```python
from build123d import *

# Parameters (mm, degrees)
SKETCH1_R           = 6.5
BOSS_EXTRUDE1_DEPTH = 8.000000002
SKETCH2_R           = 5
CUT_EXTRUDE1_DEPTH  = 5.999999938


with BuildPart() as part:
    # Sketch1 → Boss-Extrude1 (new body)
    with BuildSketch(Plane(origin=(0, 0, 0), x_dir=(1, 0, 0), z_dir=(0, 1, 0))):
        Circle(SKETCH1_R)
        with BuildLine():
            ThreePointArc((6.5, 0), (5.252972745, -3.828351779), (1.990376203, -6.187762323))
            Line((1.990376203, -6.187762323), (12.348635171, -2.855890303))
            ThreePointArc((12.348635171, -2.855890303), (14.43, 0), (12.348635171, 2.855890303))
            Line((12.348635171, 2.855890303), (1.990376203, 6.187762323))
            ThreePointArc((1.990376203, 6.187762323), (5.252972745, 3.828351779), (6.5, 0))
        make_face()
    extrude(amount=BOSS_EXTRUDE1_DEPTH)

    # Sketch2 → Cut-Extrude1 (cut)
    with BuildSketch(Plane(origin=(0, 8.000000002, 0), x_dir=(1, 0, 0), z_dir=(0, 1, 0))):
        with Locations(Location((0, 0, 0), (0, 0, 270))):
            Circle(SKETCH2_R)
    extrude(amount=-CUT_EXTRUDE1_DEPTH, mode=Mode.SUBTRACT)


solid = part.part
```
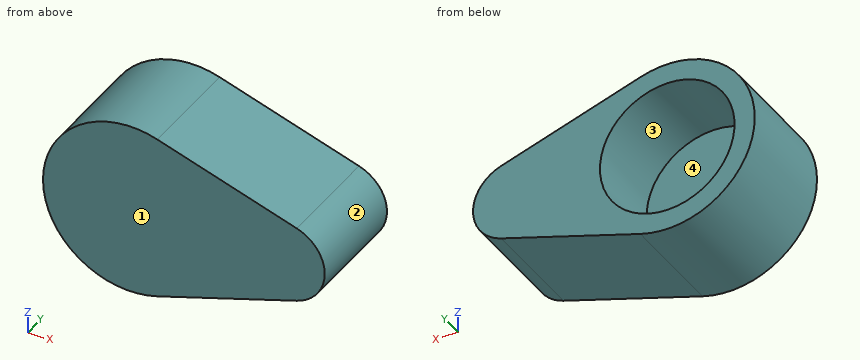
CAD build for the part. Positions are in the model's coordinates, mm. Face numbers are marked on the shaded views. Coordinates: 2 decimals unless noted, no trailing zeros. Write each loop counter-clockwise with the first axis right and the second up, starting at its lowest first coordinate (ties: lowest second). Pieces come first, ordered by that corner, then holes. Notation, with made-up numbers: (-36, 70) -> (-5, 70) arc R20 ccw to (-5, 95) -> close; hole circle Ø6 at (49.25, -26). An arc over 180 degrees is marked (long way). Return JSON: item names as keys, results as strings. Group by question number.
Q1. Flat gauge pins, fed straight in: pin 1 (1 mm diameter, centred on x = 6, z = 0.5, fed in from -Y); pin 2 (2 mm diameter, centred on x = -3, y = 4.5, fed in from +Z); pin 3 (1.5 mm diameter, centred on y = 6.5, z = -3.5, fed in from -X); pin 4 (1.5 mm diameter, centred on y = 3.5, z = 1.5, fed in from +X). Where does each tip first touch, or does it go through?
Q2. Cut at D-D, the plane z = 5.25. Give the cut face in (x, y), then the cut area to 3 significant figures.
Q3. Pull direction Z, two halves, no side cores. Call the marked faces 1, 2, 3 and 4: released by +Z, released by -Z, zero draft, split by the parting line, or undercut.
Q4. Drill centre lines: line 1 (Y direction, x = 1, z = -0.25); line 2 (X direction, y = 7.75, z = -0.25); line 3 (Z direction, x = 2.75, y = 6.25). Where is each one in solid material? Low to high.
Q5. Cut at C-C, the plane x = -3.25. Give the cut face in (y, z), then the cut area to 3 significant figures.
Q6. Cut at A-A, the plane y = 7.75. Give the cut face in (x, z).
Q7. Cut at B-B, the plane z = 0. Give the cut face in (x, y), then the cut area to 3 significant figures.
Returned:
{
 "1": {"pin 1": "stops at y = 0", "pin 2": "stops at z = 6.18", "pin 3": "stops at x = -5.89", "pin 4": "stops at x = 14.33"},
 "2": {"outline": "(-3.83, 0) -> (4.91, 0) -> (4.91, 8) -> (-3.83, 8) -> close", "area": "69.9 mm2"},
 "3": {"face 1": "zero draft", "face 2": "split by the parting line", "face 3": "undercut", "face 4": "undercut"},
 "4": {"line 1": "y = 0 to 2", "line 2": "x = -6.5 to -4.99, 4.99 to 14.42", "line 3": "z = -5.94 to -4.18, 4.18 to 5.94"},
 "5": {"outline": "(0, -5.63) -> (8, -5.63) -> (8, -3.8) -> (2, -3.8) -> (2, 3.8) -> (8, 3.8) -> (8, 5.63) -> (0, 5.63) -> close", "area": "44.5 mm2"},
 "6": {"outline": "(1.99, -6.19) -> (12.35, -2.86) arc R3 ccw to (12.35, 2.86) -> (1.99, 6.19) arc R6.5 ccw (long way) to start; hole circle Ø10 at (0, 0)"},
 "7": {"outline": "(-6.5, 0) -> (14.43, 0) -> (14.43, 8) -> (5, 8) -> (5, 2) -> (-5, 2) -> (-5, 8) -> (-6.5, 8) -> close", "area": "107 mm2"}
}
